```python
from build123d import *

# Parameters (mm, degrees)
CROQUIS1_R              = 3
SALIENTE_EXTRUIR1_DEPTH = 2.5
CROQUIS2_R              = 2.1
SALIENTE_EXTRUIR2_DEPTH = 20
CORTAR_EXTRUIR1_DEPTH   = 2.5


with BuildPart() as part:
    # Croquis1 → Saliente-Extruir1 (new body)
    with BuildSketch(Plane(origin=(0, 0, 0), x_dir=(1, 0, 0), z_dir=(0, 1, 0))):
        Circle(CROQUIS1_R)
    extrude(amount=SALIENTE_EXTRUIR1_DEPTH)

    # Croquis2 → Saliente-Extruir2 (add)
    with BuildSketch(Plane(origin=(0, 0, 0), x_dir=(1, 0, 0), z_dir=(0, 1, 0))):
        Circle(CROQUIS2_R)
    extrude(amount=-SALIENTE_EXTRUIR2_DEPTH)

    # Croquis4 → Cortar-Extruir1 (cut)
    with BuildSketch(Plane(origin=(0, 3.7, 0), x_dir=(1, 0, 0), z_dir=(0, 1, 0))):
        Polygon((1.732050808, 0), (0.866025404, 1.5), (-0.866025404, 1.5), (-1.732050808, 0), (-0.866025404, -1.5), (0.866025404, -1.5), align=None)
    extrude(amount=-CORTAR_EXTRUIR1_DEPTH, mode=Mode.SUBTRACT)


solid = part.part
```
Build history of the part. All positions in model axes, mm. A direction names the side the tool comes from. Coordinates: 2 decimals unless noted, no trailing zeros. Write each loop counter-clockwise with the first axis right and the second up, starting at its lowest first coordinate (ties: lowest second). Pieces come first, ordered by that corner, then holes.
1. Band-saw the part on B-B, the plane z = 1. Give the cut face in (x, y), and give its area (3 significant figures).
Answer block:
outline: (-2.83, 0) - (-1.85, 0) - (-1.85, -20) - (1.85, -20) - (1.85, 0) - (2.83, 0) - (2.83, 2.5) - (1.15, 2.5) - (1.15, 1.2) - (-1.15, 1.2) - (-1.15, 2.5) - (-2.83, 2.5) - close
area: 85.0 mm2
2. Band-saw the part on C-C, the plane y = -13.25. Give the cut face in (x, z).
Answer block:
outline: circle Ø4.2 at (0, 0)
3. 3-axis set-ups, long thin cutter, end or side, ignore diameter. For faces 1 (the cylindrical face through (2.003, -9.86, -0.631)), 2 (the flat face through (1.3, 2.5, 1.3)), 3 (the flat face through (-1.305, 1.859, 0.74)): which of +Z, -Z, +X, -X, +Y, -Y reach the whole face in a straight line?
Answer block:
face 1: -Y
face 2: +Z, -Z, +X, -X, +Y
face 3: +Y
4. Drill centre lines: probe 1 along Y at (x, z) = (-1.05, 0.2); probe 2 along Y at (x, z) = (2.7, 0.15); probe 3 along Z at (x, y) = (-1.2, -5.75). Where is each one in solid material? Low to high.
Answer block:
probe 1: y = -20 to 1.2
probe 2: y = 0 to 2.5
probe 3: z = -1.72 to 1.72
5. Band-saw the part on A-A, the plane x = 0. Give the cut face in (y, z), and give its area (3 significant figures).
Answer block:
outline: (-20, -2.1) - (0, -2.1) - (0, -3) - (2.5, -3) - (2.5, -1.5) - (1.2, -1.5) - (1.2, 1.5) - (2.5, 1.5) - (2.5, 3) - (0, 3) - (0, 2.1) - (-20, 2.1) - close
area: 95.1 mm2
6. Band-saw the part on D-D, the plane x = -2.3. Give the cut face in (y, z).
Answer block:
outline: (0, -1.93) - (2.5, -1.93) - (2.5, 1.93) - (0, 1.93) - close
7. Pull direction X, two halves, no side cores. Call faces 4 (the cylindrical face through (-3, 1, 0)), 5 (the flat face through (-1.293, 1.859, -0.76)), 6 (the flat face through (1.3, 0, 2)): released by +X, released by -X, zero draft, split by the parting line, or undercut.
Answer block:
face 4: split by the parting line
face 5: undercut
face 6: zero draft
8. Drop flat-ended pins along their axis: pin 1 (1.5 mm diameter, centred on x = -0.5, y = -6, fed in from +Z); pin 2 (1 mm diameter, centred on x = 0.5, y = -16.5, fed in from -Z); pin 3 (0.9 mm diameter, centred on x = 0, z = 0.5, fed in from +Y). Give the stop position or say it passes through.
Answer block:
pin 1: stops at z = 2.1
pin 2: stops at z = -2.1
pin 3: stops at y = 1.2
